```python
from build123d import *

# Parameters (mm, degrees)
SKETCH1_W           = 20
SKETCH1_H           = 127
BOSS_EXTRUDE1_DEPTH = 5
CUT_EXTRUDE1_DEPTH  = 3
SKETCH4_R           = 2.5
CUT_EXTRUDE2_DEPTH  = 3
FILLET1_R           = 5


with BuildPart() as part:
    # Sketch1 → Boss-Extrude1 (new body)
    with BuildSketch(Plane(origin=(0, 0, 0), x_dir=(1, 0, 0), z_dir=(0, 1, 0))):
        Rectangle(SKETCH1_W, SKETCH1_H)
    extrude(amount=BOSS_EXTRUDE1_DEPTH)

    # Sketch3 → Cut-Extrude1 (cut)
    with BuildSketch(Plane(origin=(0, 5, 0), x_dir=(1, 0, 0), z_dir=(0, 1, 0))):
        Polygon((3.92598183, 55.75), (1.962990915, 59.15), (-1.962990915, 59.15), (-3.92598183, 55.75), (-1.962990915, 52.35), (1.962990915, 52.35), align=None)
    cut_extrude1 = extrude(amount=-CUT_EXTRUDE1_DEPTH, mode=Mode.SUBTRACT)

    # Sketch4 → Cut-Extrude2 (cut, through all)
    with BuildSketch(Plane(origin=(0, 2, 0), x_dir=(1, 0, 0), z_dir=(0, 1, 0))):
        with Locations((0, 55.75)):
            Circle(SKETCH4_R)
    cut_extrude2 = extrude(amount=-CUT_EXTRUDE2_DEPTH, mode=Mode.SUBTRACT)

    # Mirror1: Cut-Extrude1, Cut-Extrude2 across plane
    add(cut_extrude1.mirror(Plane.XY), mode=Mode.SUBTRACT)
    add(cut_extrude2.mirror(Plane.XY), mode=Mode.SUBTRACT)

    # Fillet1
    fillet1_edges = [part.edges().sort_by_distance(p)[0] for p in [
        (10, 2.5, 63.5),
        (-10, 2.5, 63.5),
        (-10, 2.5, -63.5),
        (10, 2.5, -63.5),
    ]]
    fillet(fillet1_edges, radius=FILLET1_R)


solid = part.part
```
Source: CAD feature listing. Evaluate the final solid. Frame: model axes, mm. A direction names the side the tool comes from. Give positions to 0.01 mm unless a question says otherwise; leave off trailing zeros. Loops run counter-clockwise (first coordinate to the right, second up) from the corner with the lowest first, then second, coordinate; pieces in that order, holes last. Notation, with made-up numbers: (4, -29) -> (8, -29) arc R7 ccw to (8, -22) -> close; hole circle Ø2 at (-37.5, 40). An arc over 180 degrees is marked (long way). Use a Markdown table: item, result. Add a question column.
(1) Pull-direction query (Z, two-part tool) for faces 3 (the face through (0, 2, -63.5)), 4 (the face through (-0.5, 1, 53.3)), 5 (the face through (10, 2, 1)); classes: +Z half, -Z half, draft (parallel to the pull), parting line (faces both ways), or undercut.
(2) Ray query, line 1 (Z direction, x = 0, y = 1.1); line 2 (X direction, y = 0.6, z = -55.75); line 3 (Z direction, x = -1.75, y = 1.4). Return the intervals inside material, ascending.
(3) Access query for faces 1 (the face through (3, 2, 56)), 2 (the face through (-8.57, 2.54, -62)). Directions: +Z, -Z, +X, -X, +Y, -Y. A direction counts if a zero-diameter tool reaches every point of the face in a straight line with its end or side. Return the directions, or none.
(4) Section query A-A (y = 1). Output: boundary loops of the cut face in (x, z).
(5) Section query B-B (x = 0). Output: boundary loops of the cut face in (y, z), then the cut area to 3 significant figures.
(6) First-contact query: pin 1 Ø3 at (x, z) = (0, -55.75) entering from +Y. Flat tip, straight axial feed; report the tip coordinate or a pass-through.
Checked values:
| question | item | result |
|---|---|---|
| 1 | face 3 | -Z half |
| 1 | face 4 | undercut |
| 1 | face 5 | draft |
| 2 | line 1 | -63.5 to -58.25, -53.25 to 53.25, 58.25 to 63.5 |
| 2 | line 2 | -10 to -2.5, 2.5 to 10 |
| 2 | line 3 | -63.5 to -57.54, -53.96 to 53.96, 57.54 to 63.5 |
| 3 | face 1 | +Y |
| 3 | face 2 | -Z, -X, +Y, -Y |
| 4 | outline | (-10, -58.5) arc R5 ccw to (-5, -63.5) -> (5, -63.5) arc R5 ccw to (10, -58.5) -> (10, 58.5) arc R5 ccw to (5, 63.5) -> (-5, 63.5) arc R5 ccw to (-10, 58.5) -> close; hole circle Ø5 at (0, -55.75); hole circle Ø5 at (0, 55.75) |
| 5 | outline | (0, -63.5) -> (5, -63.5) -> (5, -59.15) -> (2, -59.15) -> (2, -58.25) -> (0, -58.25) -> close; (0, -53.25) -> (2, -53.25) -> (2, -52.35) -> (5, -52.35) -> (5, 52.35) -> (2, 52.35) -> (2, 53.25) -> (0, 53.25) -> close; (0, 58.25) -> (2, 58.25) -> (2, 59.15) -> (5, 59.15) -> (5, 63.5) -> (0, 63.5) -> close |
| 5 | area | 574 mm^2 |
| 6 | pin 1 | through |
